```python
from build123d import *

# Parameters (mm, degrees)
F0_R     = 1.6
F1_DEPTH = 7.2
F2_DEPTH = 5.5
F3_R     = 1.6
F4_DEPTH = 5.5
F5_SIZE  = 0.4


with BuildPart() as f1:
    # F0 (on Front) → F1 (new body)
    with BuildSketch(Plane.XZ):
        Polygon((-35.112121, 32.045641), (-36.966095, 34.404195), (-39.93565, 33.977883), (-41.051231, 31.193017), (-39.197257, 28.834463), (-36.227701, 29.260775), align=None)
        with Locations((-38.081676, 31.619329)):
            Circle(F0_R, mode=Mode.SUBTRACT)
        with Locations((-38.081676, 31.619329)):
            Circle(F0_R)
    extrude(amount=F1_DEPTH)

    # F0 (on Front) → F2 (join)
    with BuildSketch(Plane.XZ):
        with Locations((-38.081676, 31.619329)):
            Circle(F0_R)
    extrude(amount=-F2_DEPTH)

    # F3 (on face) → F4 (join)
    with BuildSketch(Plane.XZ.offset(7.2)):
        with Locations((-38.081676, 31.619329)):
            Circle(F3_R)
    extrude(amount=F4_DEPTH)

    # F5
    f5_edges = [f1.edges().sort_by_distance(p)[0] for p in [
        (-39.681676, 5.5, 31.619329),
        (-39.681676, -12.7, 31.619329),
    ]]
    chamfer(f5_edges, length=F5_SIZE)


solid = f1.part
```
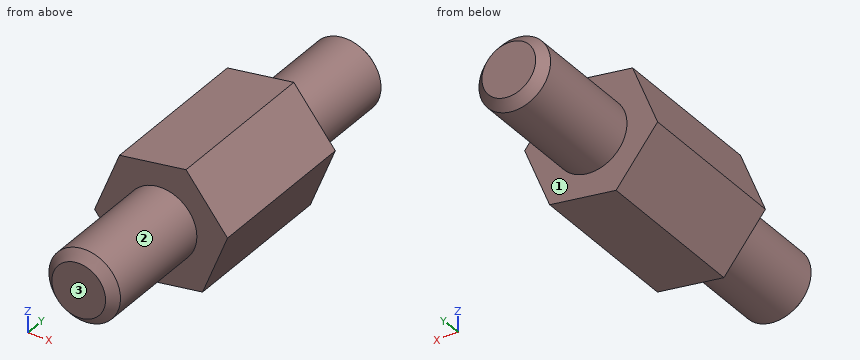
Work out the finished part from the listing and answer in its coordinate system (mm). Face numbers are marked on the shaded views. A direction names the side the tool comes from. Give positions to 0.01 mm unless a question says otherwise; leave off trailing zeros. Loops run counter-clockwise (first coordinate to the right, second up) from the corner with the lowest first, then second, coordinate; pieces in that order, holes last. Notation, with made-up numbers: (-7.5, 33) -> (23.5, 33) arc R25 ccw to (23.5, 61) -> close; hole circle Ø11 at (87.5, 72). An arc over 180 degrees is marked (long way). Write item = value, one per line. Start each with the question number.
(1) Find section B-B on x = -40.1. Give the vertices of the cut face in (y, z).
(2) Given pin 1 Ø1.5 at (y, z) = (2.5, 33) entering from +X; pin 2 Ø1.5 at (x, y) = (-36.5, -8) entering from +Z; pin 3 Ø1.5 at (x, y) = (-36.5, 2) entering from -Z, each flat-ended and moving along its own axis, determine where each tip first touches the part or whether it passes through.
(3) Find section C-C on z = 29.6. Give the vertices of the cut face in (x, y).
(4) Find section A-A on y = -0.75. Give the vertices of the cut face in (x, z), and give its area (3 significant figures).
(5) Find section D-D on y = -10. Give the vertices of the cut face in (x, z).
(6) Find the intervals of material crossed by probe 1 along Y at (x, z) = (-40, 32.8); probe 2 along X at (y, z) = (0.25, 33); probe 3 along X at (y, z) = (-9.5, 31.9), in increasing order. Write a range as from..to.
(7) Which of the six approach directions +Z, -Z, +X, -X, +Y, -Y give full straight-line access (tool end or side, diameter ignored) to the marked faces 1, 2 and 3?
From the geometry:
q1.outline = (-7.2, 29.98) -> (0, 29.98) -> (0, 33.57) -> (-7.2, 33.57) -> close
q2.pin_1 = -36.61
q2.pin_2 = 32.99
q2.pin_3 = 30.25
q3.outline = (-39.8, -7.2) -> (-36.09, -7.2) -> (-36.09, 0) -> (-39.8, 0) -> close
q4.outline = (-41.05, 31.19) -> (-39.2, 28.83) -> (-36.23, 29.26) -> (-35.11, 32.05) -> (-36.97, 34.4) -> (-39.94, 33.98) -> close
q4.area = 23.4 mm^2
q5.outline = circle Ø3.2 at (-38.08, 31.62)
q6.probe_1 = -7.2..0
q6.probe_2 = -38.89..-37.27
q6.probe_3 = -39.66..-36.51
q7.face_1 = +Y
q7.face_2 = -Y
q7.face_3 = +Z, -Z, +X, -X, -Y
